Autodesk Inventor part; units mm, degrees
ref_plane "YZ Plane" through (0, 0, 0) normal (1, 0, 0) x (0, 1, 0)
ref_plane "XZ Plane" through (0, 0, 0) normal (0, 1, 0) x (-1, 0, 0)
ref_plane "XY Plane" through (0, 0, 0) normal (0, 0, 1) x (1, 0, 0)
sketch "Skizze1" plane through (0, 0, 0) normal (1, 0, 0) x (0, 1, 0)
  arc A0 (-7.5, 0) -> (7.5, 0) centre (0, 0) ccw
  line L0 (-7.5, 0) -> (-10, 0)
  line L1 (-10, 0) -> (-10, -10)
  line L2 (-10, -10) -> (10, -10)
  line L3 (10, -10) -> (10, 0)
  line L4 (0, -12) -> (0, 2)
  line L5 (7.5, 0) -> (10, 0)
  line L6 (-14, 0) -> (14, 0)
  dimension "d0" = 20
  dimension "d1" = 7.5
  dimension "d2" = 10
extrude "Extrusion1" add sketch "Skizze1" along normal blind 300 contours A0 L4 L2 L1 L0 | A0 L5 L3 L2 L4
properties part number "Gerade_1"
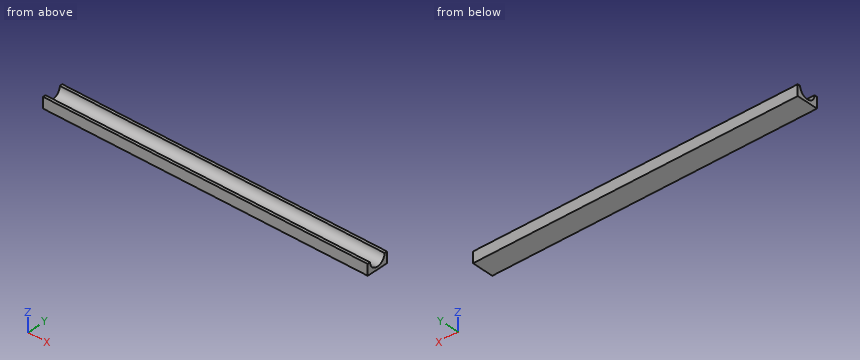
The model under review builds one solid part; all positions refer to its coordinate system, in mm. Round coordinates to 2 decimals unless told otherwise and drop trailing zeros. Write each loop counter-clockwise with the first axis right and the second up, starting at its lowest first coordinate (ties: lowest second). Pieces come first, ordered by that corner, then holes. Notation, with made-up numbers: (41.25, -24.5) - (47.25, -24.5) arc R19 cw to (47.25, 9.5) - close; hole circle Ø8 at (51.5, 19.25). An arc over 180 degrees is marked (long way). One line per item, written item: value. Start each with the question number.
1. Clearance check with a flat-ended pin moving along its axis: P1, Ø12, axis at x = 122, y = 4.5, coming from the +Z side. State where the tip first meets the part, or that it passes through.
2. To check wall thickness, follow L1, parallel to Y at x = 67, z = -0.75; L2, parallel to Y at x = 202, z = -6.75; L3, parallel to Z at x = 110, y = 0.5. State the ranges of each line that lie inside material, in increasing order. Write a range as from..to.
3. Consider section B-B on y = 0. Write out the cut boundary in (x, z), and give its area (3 significant figures).
4. Consider section A-A on x = 249. Write out the cut boundary in (y, z).
Checks:
1. P1: stops at z = 0
2. L1: y = -10..-7.46, 7.46..10
2. L2: y = -10..-3.27, 3.27..10
2. L3: z = -10..-7.48
3. outline: (0, -10) - (300, -10) - (300, -7.5) - (0, -7.5) - close
3. area: 750 mm^2
4. outline: (-10, -10) - (10, -10) - (10, 0) - (7.5, 0) arc R7.5 cw to (-7.5, 0) - (-10, 0) - close
